Could you check a few things on this model? Use its own coordinates, in mm. A direction names the side the tool comes from. Coordinates: 2 decimals unless noted, no trailing zeros. Order: outer loops, then holes, each group sorted by start corner. A loop starts at its lowest first (then second) coordinate and runs counter-clockwise, first axis right, second up. Notation, with made-up numbers: (4.25, 45.5) -> (50.25, 45.5) arc R16 cw to (50.25, 49.5) -> close; hole circle Ø6 at (-16.75, 6). An arc over 180 degrees is marked (long way). Use a Markdown table: item, result. Add a question column.
1) Which directions (+Z, -Z, +X, -X, +Y, -Y) give clear straight access to the entire face, cutting with the end or side of a thin tool? Please do faces 1 (the flat face through (32, -7, 0)), 2 (the flat face through (-33.37, 34.15, 2.46)), 3 (the flat face through (-12.833, 46.036, 2.465)).
2) If we section it at B-B (z = 2.85): Write out the boundary of the cut face in (x, y).
3) If we section it at C-C (x = 91): Write out the boundary of the cut face in (y, z).
4) If we section it at A-A (y = 37.5): Write out the boundary of the cut face in (x, z), plus the area to 3 significant figures.
5) Will this pin go through, and if not, where does the flat tip stop? pin 1 Ø1 at (y, z) = (-25.5, 2.5) entering from -X.
6) If we section it at D-D (y = 0): Write out the boundary of the cut face in (x, z).
7) If I drill on L1, parallel to Y at x = 116, z = 1.05; L2, parallel to X at y = 37, z = 3.7; L3, parallel to Y at x = 100.5, z = 4.15, over which ranges is the centre line in solid material (lowest first)? Write a range as [from, to].
8) Thinking about a two-plate mould opening in X: for faces 4 (the flat face through (32, -7, 5)), 5 (the cylindrical face through (19.2, 28.3, 2.5)), 6 (the flat face through (-44.89, -37.75, 2.46)), which applies, +X half, -X half, draft (parallel to the pull), parting line (faces both ways), or undercut?
```python
from build123d import *

# Parameters (mm, degrees)
BOSS_EXTRUDE2_DEPTH = 5


with BuildPart() as part:
    # Sketch1 → Boss-Extrude2 (new body)
    with BuildSketch(Plane.XY):
        with BuildLine():
            Line((-30.410051578, 28.86238305), (-36.410051578, 39.588721298))
            ThreePointArc((-36.410051578, 39.588721298), (-42.759129148, 31.880332669), (-41.076365657, 22.036636805))
            ThreePointArc((-41.076365657, 22.036636805), (-38.658640478, 3.297393101), (-50.044050262, -11.781635174))
            ThreePointArc((-50.044050262, -11.781635174), (-59.820088495, -29.100692514), (-49.820508076, -46.291651246))
            Line((-49.820508076, -46.291651246), (-39.820508076, -28.97114317))
            ThreePointArc((-39.820508076, -28.97114317), (-12.5, -21.650635095), (-5.179491924, -48.97114317))
            ThreePointArc((-5.179491924, -48.97114317), (-5.422797128, -49.381193221), (-5.675808094, -49.78532676))
            Line((-5.675808094, -49.78532676), (-15.589541975, -66.048346043))
            ThreePointArc((-15.589541975, -66.048346043), (1.883571693, -67.682453449), (13.918479383, -54.909787119))
            ThreePointArc((13.918479383, -54.909787119), (30.208282334, -32.034409255), (56.888914824, -23.271736004))
            Line((56.888914824, -23.271736004), (115, -12))
            ThreePointArc((115, -12), (127, 0), (115, 12))
            Line((115, 12), (43.874557006, 21.783515632))
            ThreePointArc((43.874557006, 21.783515632), (18.891003915, 28.477838507), (0.601773699, 46.767068722))
            ThreePointArc((0.601773699, 46.767068722), (-6.684702605, 52.358178638), (-15.790531146, 51.159373568))
            Line((-15.790531146, 51.159373568), (-9.790531146, 40.767068722))
            ThreePointArc((-9.790531146, 40.767068722), (-14.147948526, 24.50496567), (-30.410051578, 28.86238305))
        make_face()
    extrude(amount=BOSS_EXTRUDE2_DEPTH)


solid = part.part
```
Answer sheet:
| question | item | result |
|---|---|---|
| 1 | face 1 | -Z, +X, -X, +Y, -Y |
| 1 | face 2 | +Z, -Z, +Y |
| 1 | face 3 | +Z, -Z, -X |
| 2 | outline | (-50.04, -11.78) arc R20 ccw to (-49.82, -46.29) -> (-39.82, -28.97) arc R20 cw to (-5.18, -48.97) arc R20 cw to (-5.68, -49.79) -> (-15.59, -66.05) arc R20 ccw to (13.92, -54.91) arc R45 cw to (56.89, -23.27) -> (115, -12) arc R12 ccw to (115, 12) -> (43.87, 21.78) arc R49.97 cw to (0.6, 46.77) arc R12 ccw to (-15.79, 51.16) -> (-9.79, 40.77) arc R11.9 cw to (-30.41, 28.86) -> (-36.41, 39.59) arc R12 ccw to (-41.08, 22.04) arc R25 cw to start |
| 3 | outline | (-16.66, 0) -> (15.3, 0) -> (15.3, 5) -> (-16.66, 5) -> close |
| 4 | outline | (-39.42, 0) -> (-35.24, 0) -> (-35.24, 5) -> (-39.42, 5) -> close; (-8.5, 0) -> (7.49, 0) -> (7.49, 5) -> (-8.5, 5) -> close |
| 4 | area | 101 mm2 |
| 5 | pin 1 | x = -59.6 |
| 6 | outline | (-39.78, 0) -> (127, 0) -> (127, 5) -> (-39.78, 5) -> close |
| 7 | L1 | [-11.96, 11.96] |
| 7 | L2 | [-39.92, -34.96], [-8.4, 7.97] |
| 7 | L3 | [-14.81, 13.99] |
| 8 | face 4 | draft |
| 8 | face 5 | +X half |
| 8 | face 6 | undercut |
